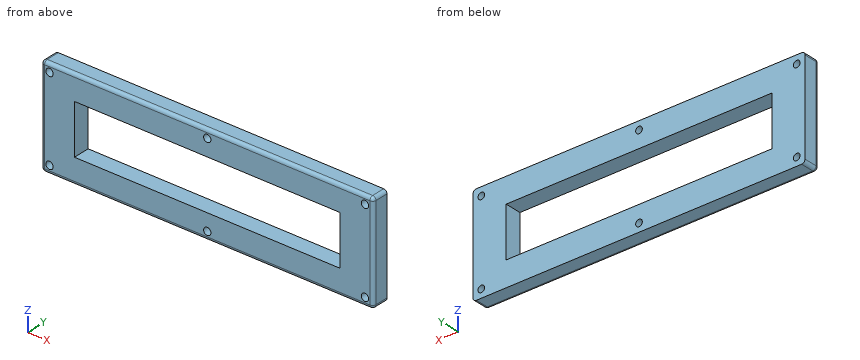
Solid Edge part; units mm, degrees
sketch "Sketch1" plane through (0, 0, 0) normal (0, -1, 0) x (1, 0, 0)
  line L0 (50, 15) -> (-50, 15)
  line L1 (-50, 15) -> (-50, -15)
  line L2 (-50, -15) -> (50, -15)
  line L3 (50, -15) -> (50, 15)
extrude "Protrusion1" add sketch "Sketch1" against normal blind 5
sketch "Sketch2" plane through (0, 0, 0) normal (0, -1, 0) x (1, 0, 0)
  circle A0 centre (47.5, 12.5) radius 1
  circle A1 centre (-47.5, 12.5) radius 1
  circle A2 centre (-47.5, -12.5) radius 1
  circle A3 centre (47.5, -12.5) radius 1
  circle A4 centre (0, -12.5) radius 1
  circle A5 centre (0, 12.5) radius 1
extrude "ExtrudedCutout_1" cut sketch "Sketch2" against normal blind 5
sketch "Sketch3" plane through (0, 0, 0) normal (0, -1, 0) x (1, 0, 0)
  circle A0 centre (47.5, 12.5) radius 1.1
  circle A1 centre (-47.5, 12.5) radius 1.1
  circle A2 centre (-47.5, -12.5) radius 1.1
  circle A3 centre (47.5, -12.5) radius 1.1
  circle A4 centre (0, 12.5) radius 1.1
  circle A5 centre (0, -12.5) radius 1.1
extrude "ExtrudedCutout_2" cut sketch "Sketch3" against normal blind 2.5
fillet "Round_1" radius 1 8 edges at (50, 2.5, 15) (50, 0, 0) (0, 0, 15) (50, 2.5, -15) (0, 0, -15) (-50, 2.5, -15) (-50, 0, 0) (-50, 2.5, 15)
sketch "Sketch4" plane through (0, 0, 0) normal (0, -1, 0) x (-1, 0, 0)
  line L0 (-40, -7.5) -> (40, -7.5)
  line L1 (40, -7.5) -> (40, 7.5)
  line L2 (40, 7.5) -> (-40, 7.5)
  line L3 (-40, 7.5) -> (-40, -7.5)
extrude "ExtrudedCutout_3" cut sketch "Sketch4" against normal blind 5
Geometry: final body of the model. Coordinates: model frame, mm. Round coordinates to 2 decimals unless told otherwise and drop trailing zeros. Loops run counter-clockwise (first coordinate to the right, second up) from the corner with the lowest first, then second, coordinate; pieces in that order, holes last. Notation, with made-up numbers: (-31, -32.5) -> (1, -32.5) arc R18 ccw to (1, -18.5) -> close; hole circle Ø2 at (-7.5, 88.5). An arc over 180 degrees is marked (long way). Use one line per item in the form item = value. Start each with the question number.
1) Section C-C on x = -18.5. Output: boundary loops of the cut face in (y, z), then the cut area to 3 significant figures.
2) Line query: L1, parallel to Z at x = 0, y = 3.1; L2, parallel to Z at x = -47.5, y = 3.15; L3, parallel to Z at x = 11, y = 3.3. Output: solid intervals per line, ascending.
3) Section B-B on x = -47.5. Output: boundary loops of the cut face in (y, z).
4) Section A-A on z = 12.5. Give the number of separate pieces and of enclosed holes in the cut face, then the cut area to 3 significant figures.
5) Section D-D on y = 3.65. Output: boundary loops of the cut face in (x, z).
6) First-contact query: P1, Ø4, axis at x = -34, z = 7, coming from the -Y side; P2, Ø1.8, axis at x = 0, z = 12.5, coming from the -Y side. Flat tips, straight axial feed; report the tip coordinate or a pass-through.
Response:
q1.outline = (0, -14) arc R1 ccw to (1, -15) -> (5, -15) -> (5, -7.5) -> (0, -7.5) -> close; (0, 7.5) -> (5, 7.5) -> (5, 15) -> (1, 15) arc R1 ccw to (0, 14) -> close
q1.area = 74.6 mm^2
q2.L1 = -15 to -13.5, -11.5 to -7.5, 7.5 to 11.5, 13.5 to 15
q2.L2 = -15 to -13.5, -11.5 to 11.5, 13.5 to 15
q2.L3 = -15 to -7.5, 7.5 to 15
q3.outline = (0, -14) arc R1 ccw to (1, -15) -> (5, -15) -> (5, -13.5) -> (2.5, -13.5) -> (2.5, -13.6) -> (0, -13.6) -> close; (0, -11.4) -> (2.5, -11.4) -> (2.5, -11.5) -> (5, -11.5) -> (5, 11.5) -> (2.5, 11.5) -> (2.5, 11.4) -> (0, 11.4) -> close; (0, 13.6) -> (2.5, 13.6) -> (2.5, 13.5) -> (5, 13.5) -> (5, 15) -> (1, 15) arc R1 ccw to (0, 14) -> close
q4.separate_pieces = 4
q4.enclosed_holes = 0
q4.area = 468 mm^2
q5.outline = (-50, -14) arc R1 ccw to (-49, -15) -> (49, -15) arc R1 ccw to (50, -14) -> (50, 14) arc R1 ccw to (49, 15) -> (-49, 15) arc R1 ccw to (-50, 14) -> close; hole circle Ø2 at (-47.5, -12.5); hole circle Ø2 at (-47.5, 12.5); hole (-40, -7.5) -> (40, -7.5) -> (40, 7.5) -> (-40, 7.5) -> close; hole circle Ø2 at (0, -12.5); hole circle Ø2 at (0, 12.5); hole circle Ø2 at (47.5, -12.5); hole circle Ø2 at (47.5, 12.5)
q6.P1 = 0
q6.P2 = through
